Read the model definition and answer for the solid it produces. Units are mm, in the model's axes. Round coordinates to 2 decimals unless told otherwise and drop trailing zeros. Loops run counter-clockwise (first coordinate to the right, second up) from the corner with the lowest first, then second, coordinate; pieces in that order, holes last. Notation, with made-up numbers: (68.5, 7.25) - (107.5, 7.25) arc R19 ccw to (107.5, 18.25) - close; hole circle Ø3 at (-15, -25). An arc over 180 degrees is marked (long way). Answer as CSV lines item,"result".
```python
from build123d import *

# Parameters (mm, degrees)
SKETCH1_W                 = 370
SKETCH1_H                 = 40
BOSS_EXTRUDE1_DEPTH       = 4
CUT_EXTRUDE1_REACH        = 188.121
SKETCH2_R                 = 10.5
SKETCH2_R_2               = 5.5
M4X0_7_TAPPED_HOLE1_D     = 3.3
M4X0_7_TAPPED_HOLE1_DEPTH = 4
CHAMFER1_SIZE             = 3
FILLET1_R                 = 3
M3X0_5_TAPPED_HOLE1_D     = 2.5


with BuildPart() as part:
    # Sketch1 → Boss-Extrude1 (new body)
    with BuildSketch(Plane(origin=(0, 0, 0), x_dir=(1, 0, 0), z_dir=(0, 1, 0))):
        Rectangle(SKETCH1_W, SKETCH1_H)
    extrude(amount=BOSS_EXTRUDE1_DEPTH)

    # Sketch2 → Cut-Extrude1 (cut, up to next)
    with BuildSketch(Plane(origin=(0, 4, 0), x_dir=(1, 0, 0), z_dir=(0, 1, 0)), mode=Mode.PRIVATE) as cut_extrude1_sk1:
        with Locations(Location((165, 5, 0), (0, 0, 270))):
            Circle(SKETCH2_R)
    cut_extrude1_tool1 = extrude(cut_extrude1_sk1.sketch, amount=-CUT_EXTRUDE1_REACH, mode=Mode.PRIVATE) & part.part
    # Sketch2 → Cut-Extrude1 (cut, up to next)
    with BuildSketch(Plane(origin=(0, 4, 0), x_dir=(1, 0, 0), z_dir=(0, 1, 0)), mode=Mode.PRIVATE) as cut_extrude1_sk2:
        with Locations(Location((-165, 5, 0), (0, 0, 270))):
            Circle(SKETCH2_R)
    cut_extrude1_tool2 = extrude(cut_extrude1_sk2.sketch, amount=-CUT_EXTRUDE1_REACH, mode=Mode.PRIVATE) & part.part
    # Sketch2 → Cut-Extrude1 (cut, up to next)
    with BuildSketch(Plane(origin=(0, 4, 0), x_dir=(1, 0, 0), z_dir=(0, 1, 0)), mode=Mode.PRIVATE) as cut_extrude1_sk3:
        with Locations(Location((0, 4, 0), (0, 0, 270))):
            Circle(SKETCH2_R_2)
    cut_extrude1_tool3 = extrude(cut_extrude1_sk3.sketch, amount=-CUT_EXTRUDE1_REACH, mode=Mode.PRIVATE) & part.part
    add(cut_extrude1_tool1.solids().sort_by_distance((165, 4, -5))[0], mode=Mode.SUBTRACT)
    add(cut_extrude1_tool2.solids().sort_by_distance((-165, 4, -5))[0], mode=Mode.SUBTRACT)
    add(cut_extrude1_tool3.solids().sort_by_distance((0, 4, -4))[0], mode=Mode.SUBTRACT)

    # M4x0.7 Tapped Hole1
    with Locations(Plane(origin=(0, 4, 0), x_dir=(1, 0, 0), z_dir=(0, 1, 0))):
        with Locations((175, 2), (155, 15), (175, 15), (155, -5), (175, -5), (-175, 15), (-155, 15), (-175, -5), (-155, -5), (-140, 8.394191797), (-140, -7.610688145), (140, 8.394191797), (140, -7.610688145)):
            Hole(M4X0_7_TAPPED_HOLE1_D / 2, depth=M4X0_7_TAPPED_HOLE1_DEPTH)

    # Chamfer1
    chamfer1_edges = [part.edges().sort_by_distance(p)[0] for p in [
        (185, 2, 20),
        (-185, 2, 20),
    ]]
    chamfer(chamfer1_edges, length=CHAMFER1_SIZE)

    # Fillet1
    fillet1_edges = [part.edges().sort_by_distance(p)[0] for p in [
        (-185, 2, -20),
        (185, 2, -20),
    ]]
    fillet(fillet1_edges, radius=FILLET1_R)

    # M3x0.5 Tapped Hole1 (through all)
    with Locations(Plane(origin=(0, 4, 0), x_dir=(1, 0, 0), z_dir=(0, 1, 0))):
        with Locations((0, 12.1), (8.1, 4), (0, -4.1), (-8.1, 4)):
            Hole(M3X0_5_TAPPED_HOLE1_D / 2)


solid = part.part
```
1) A cutting plane is placed at A-A, the plane x = -165. Determine the outline of the cut face in (y, z), plus the area to 3 significant figures.
Entries:
outline,"(0, -20) - (4, -20) - (4, -15.5) - (0, -15.5) - close; (0, 5.5) - (4, 5.5) - (4, 20) - (0, 20) - close"
area,"76.0 mm^2"
2) Find the intervals of material crossed by line 1 (X direction, y = 3.65, z = 8); line 2 (Z direction, x = -140, y = 3.25); line 3 (Z direction, x = 8.1, y = 2.55), in increasing order.
Entries:
line 1,"x = -185 to -141.6, -138.4 to 138.4, 141.6 to 185"
line 2,"z = -20 to -10.04, -6.74 to 5.96, 9.26 to 20"
line 3,"z = -20 to -5.25, -2.75 to 20"
3) The mould has two halves that part along Z. Classify faces 1 (the face through (-3, 4, 4)), 2 (the face through (155.078, 2.028, -8.435)): pulls with the +Z half, pulls with the -Z half, needs draft (parallel to the pull), parting line crosses it, or undercut.
Entries:
face 1,"needs draft"
face 2,"undercut"
4) A cutting plane is placed at B-B, the plane y = 2. Count the separate pieces of the cut face and the enclosed holes in it, plus the area to 3 significant figures.
Entries:
separate pieces,"1"
enclosed holes,"19"
area,"13,900 mm^2"
